CAD build for the part. Positions are in the model's coordinates, mm. A direction names the side the tool comes from. Round coordinates to 2 decimals unless told otherwise and drop trailing zeros. Loops run counter-clockwise (first coordinate to the right, second up) from the corner with the lowest first, then second, coordinate; pieces in that order, holes last.
```python
from build123d import *

# Parameters (mm, degrees)
SKETCH1_W           = 85
SKETCH1_H           = 150
BOSS_EXTRUDE1_DEPTH = 18
SKETCH2_W           = 30
SKETCH2_H           = 150
BOSS_EXTRUDE2_DEPTH = 82
SKETCH3_W           = 55
SKETCH3_H           = 74
BOSS_EXTRUDE3_DEPTH = 45
CUT_EXTRUDE1_DEPTH  = 74
SKETCH5_W           = 85
SKETCH5_H           = 36
BOSS_EXTRUDE4_DEPTH = 26
SKETCH7_W           = 150
SKETCH7_H           = 37
CUT_EXTRUDE2_DEPTH  = 10
BOSS_EXTRUDE5_DEPTH = 10


with BuildPart() as part:
    # Sketch1 → Boss-Extrude1 (new body)
    with BuildSketch(Plane(origin=(0, 0, 0), x_dir=(1, 0, 0), z_dir=(0, 1, 0))):
        with Locations((3.434439448, 45.309233449)):
            Rectangle(SKETCH1_W, SKETCH1_H)
    extrude(amount=BOSS_EXTRUDE1_DEPTH)

    # Sketch2 → Boss-Extrude2 (add)
    with BuildSketch(Plane(origin=(0, 18, 0), x_dir=(1, 0, 0), z_dir=(0, 1, 0))):
        with Locations((-24.065560552, 45.309233449)):
            Rectangle(SKETCH2_W, SKETCH2_H)
    extrude(amount=BOSS_EXTRUDE2_DEPTH)

    # Sketch3 → Boss-Extrude3 (add)
    with BuildSketch(Plane(origin=(0, 18, 0), x_dir=(1, 0, 0), z_dir=(0, 1, 0))):
        with Locations((18.434439448, 45.309233449)):
            Rectangle(SKETCH3_W, SKETCH3_H)
    extrude(amount=BOSS_EXTRUDE3_DEPTH)

    # Sketch4 → Cut-Extrude1 (cut)
    with BuildSketch(Plane.XY.offset(-8.309233449)):
        Polygon((45.934439448, 18), (-9.065560552, 63), (45.934439448, 63), align=None)
    extrude(amount=-CUT_EXTRUDE1_DEPTH, mode=Mode.SUBTRACT)

    # Sketch5 → Boss-Extrude4 (add)
    with BuildSketch(Plane(origin=(0, 18, 0), x_dir=(1, 0, 0), z_dir=(0, 1, 0))):
        with Locations((3.434439448, 45.309233449)):
            Rectangle(SKETCH5_W, SKETCH5_H)
    extrude(amount=BOSS_EXTRUDE4_DEPTH)

    # Sketch7 → Cut-Extrude2 (cut)
    with BuildSketch(Plane(origin=(-9.065560552, 0, 0), x_dir=(0, 0, -1), z_dir=(1, 0, 0))):
        with Locations((45.309233449, 81.5)):
            Rectangle(SKETCH7_W, SKETCH7_H)
    extrude(amount=-CUT_EXTRUDE2_DEPTH, mode=Mode.SUBTRACT)

    # Sketch8 → Boss-Extrude5 (add)
    with BuildSketch(Plane(origin=(-19.065560552, 0, 0), x_dir=(0, 0, -1), z_dir=(1, 0, 0))):
        Polygon((2.809233449, 100), (87.809233449, 100), (120.309233449, 63), (-29.690766551, 63), align=None)
    extrude(amount=BOSS_EXTRUDE5_DEPTH)


solid = part.part
```
Item 1: Two-plate mould, pull along Z, no slides. Class faces 1 (the flat face through (-9.066, 69, -46)), 2 (the flat face through (37, 37, -63.309)), 3 (the flat face through (37, 37, -27.309)): released by +Z, released by -Z, zero draft, split by the parting line, or undercut.
Answers follow:
face 1: zero draft
face 2: released by -Z
face 3: released by +Z
Item 2: 3-axis set-ups, long thin cutter, end or side, ignore diameter. For faces 4 (the flat face through (30, 44, -46)), 5 (the flat face through (-14.14, 81.76, -103.83)), 6 (the flat face through (12, 35, -8.309)): which of +Z, -Z, +X, -X, +Y, -Y reach the whole face in a straight line?
Answers follow:
face 4: +Z, -Z, +X, +Y
face 5: -Z, +X, +Y
face 6: +Z, +X, +Y
Item 3: Probe line 1 (X direction, y = 60, z = -110.5); line 2 (Z direction, x = 42.5, y = 25.5); line 3 (Y direction, x = 42.5, z = -6). List the from-to ranges inside material, lowest first.
Answers follow:
line 1: x = -39.07 to -9.07
line 2: z = -63.31 to -27.31
line 3: y = 0 to 18
Item 4: Cut at C-C, the plane x = 33. Give the cut face in (y, z).
Answers follow:
outline: (0, -120.31) - (18, -120.31) - (18, -82.31) - (28.58, -82.31) - (28.58, -63.31) - (44, -63.31) - (44, -27.31) - (28.58, -27.31) - (28.58, -8.31) - (18, -8.31) - (18, 29.69) - (0, 29.69) - close
Item 5: Flat gauge pins, fed straight in: P1, Ø12, axis at y = 61, z = -41, coming from the +X side; P2, Ø11.5, axis at x = 21.5, z = -105.5, coming from the +Y side; P3, Ø16, axis at y = 84.5, z = 14.5, coming from the +X side. Where does each tip first touch, or does it go through?
Answers follow:
P1: stops at x = 0.71
P2: stops at y = 18
P3: stops at x = -9.07
Item 6: Cut at B-B, the plane y = 34.5. Give the cut face in (x, z), plus the area to 3 significant figures.
Answers follow:
outline: (-39.07, -120.31) - (-9.07, -120.31) - (-9.07, -82.31) - (25.77, -82.31) - (25.77, -63.31) - (45.93, -63.31) - (45.93, -27.31) - (25.77, -27.31) - (25.77, -8.31) - (-9.07, -8.31) - (-9.07, 29.69) - (-39.07, 29.69) - close
area: 7,800 mm2
Item 7: Cut at D-D, the plane y = 85. Give the cut face in (x, z), plus the area to 3 significant figures.
Answers follow:
outline: (-39.07, -120.31) - (-19.07, -120.31) - (-19.07, -100.98) - (-9.07, -100.98) - (-9.07, 10.37) - (-19.07, 10.37) - (-19.07, 29.69) - (-39.07, 29.69) - close
area: 4,110 mm2
Item 8: Cut at A-A, the plane z = -60.5. Give the cut face in (x, y).
Answers follow:
outline: (-39.07, 0) - (45.93, 0) - (45.93, 44) - (14.16, 44) - (-9.07, 63) - (-9.07, 100) - (-39.07, 100) - close
